Geometry: see drawing. Coordinates: mm, zero at the bounding-box minimum. A direction names the side the tool comes from. Coordinates: 2 decimals unless noted, no trailing zeros. Write each loop counter-clockwise with the first axis right and the second up, starting at its lowest first coordinate (ties: lowest second). Pieces come first, ordered by that corner, then holes.
1) Section query B-B (z = 16.5). Output: boundary loops of the cut face in (x, y) (3 decimals), then the cut area to 3 significant figures.
2) Section query A-A (z = 13). Output: boundary loops of the cut face in (x, y) (3 decimals), then the cut area to 3 significant figures.
3) Set-up query: the marked faces 1 and 2. Return all of +Z, -Z, +X, -X, +Y, -Y with unobstructed straight access to the full face (end or side cutting, diameter ignored); none if empty.
4) Line query: L1, parallel to Y at x = 2.45, z = 6.75; L2, parallel to Y at x = 3.6, z = 9.5; L3, parallel to X at y = 3.85, z = 4.75. Output: solid intervals per line, ascending.
5) Pin query (flat end, axial travel): pin 1 Ø1.5 at (x, y) = (1, 2.5) entering from -Z; pin 2 Ø2 at (y, z) = (1.5, 14) entering from -X (3 decimals). Return the tip coordinate at first contact, or that it passes through.
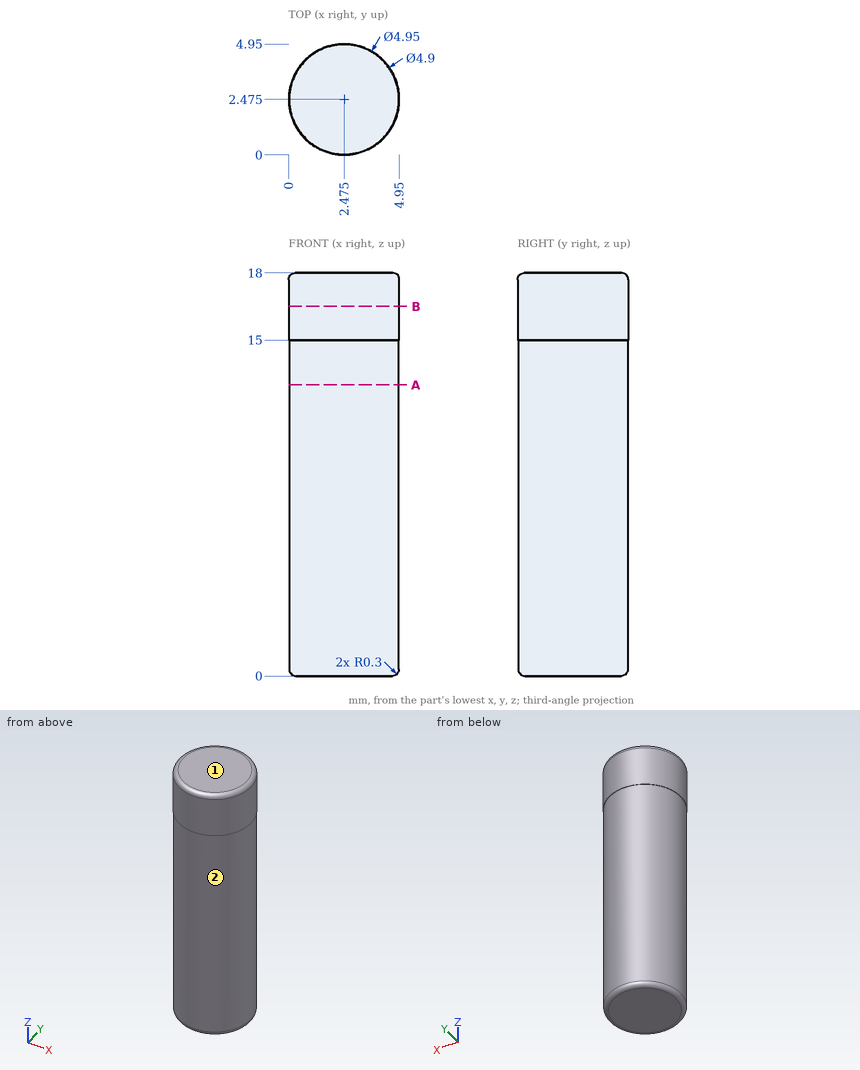
Answer:
1. outline: circle Ø4.95 at (2.475, 2.475)
1. area: 19.2 mm2
2. outline: circle Ø4.9 at (2.475, 2.475)
2. area: 18.9 mm2
3. face 1: +Z, +X, -X, +Y, -Y
3. face 2: -Z
4. L1: y = 0.03 to 4.92
4. L2: y = 0.3 to 4.65
4. L3: x = 0.45 to 4.5
5. pin 1: stops at z = 0
5. pin 2: stops at x = 0.025
